Can you work these out from the model? Positions are in its coordinate system, mm. Give positions to 0.01 mm unless a question says otherwise; leave off trailing zeros. Order: outer loops, then holes, each group sorted by start corner. A loop starts at its lowest first (then second) coordinate and runs counter-clockwise, first axis right, second up.
Item 1: I want a section at B-B, the plane z = 3. Write out the boundary of the cut face in (x, y), then the cut area to 3 significant figures.
Item 2: If I drill on line 1 along Z through (x, y) = (0, -15) (3 decimals); line 2 along X through (y, z) = (-9, 9.5); line 3 along Z through (x, y) = (1.5, -6.5) (3 decimals), over which ranges is the centre line in solid material (lowest first)?
Item 3: I want a section at A-A, the plane y = -15. Write out the boundary of the cut face in (x, z) (1 decimal).
Item 4: I want a section at C-C, the plane x = 2. Write out the boundary of the cut face in (y, z) (3 decimals).
Item 5: I'm going to push flat-ended pins straight in: pin 1 Ø3 at (x, z) = (-11, 10) entering from +Y; pin 2 Ø10 at (x, z) = (0, 10.795) entering from -Y. Where does each tip first touch, or does it pass through?
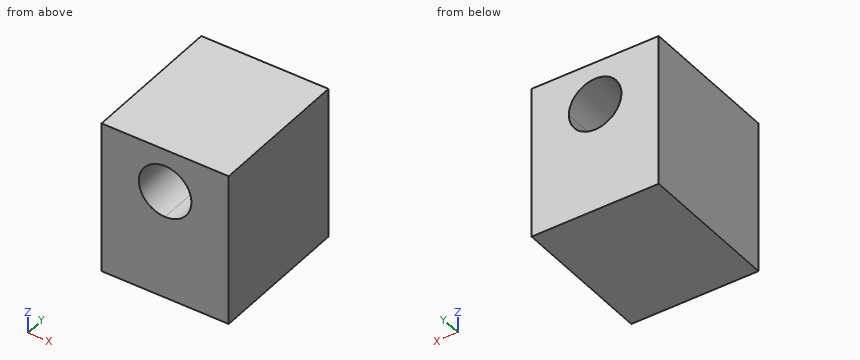
```python
from build123d import *

# Parameters (mm, degrees)
F0_W     = 41.275
F0_H     = 49.53
F1_DEPTH = 46.99


with BuildPart() as f1:
    # F0 (on Front) → F1 (new body)
    with BuildSketch(Plane.XZ):
        Rectangle(F0_W, F0_H)
        with BuildLine():
            ThreePointArc((0, 2.266854), (-6.03031, 16.82531), (8.528146, 10.795))
            ThreePointArc((8.528146, 10.795), (6.03031, 4.76469), (0, 2.266854))
        make_face(mode=Mode.SUBTRACT)
    extrude(amount=F1_DEPTH)


solid = f1.part
```
Results list:
1. outline: (-20.64, -46.99) - (-3.46, -46.99) - (-3.46, 0) - (-20.64, 0) - close; (3.46, -46.99) - (20.64, -46.99) - (20.64, 0) - (3.46, 0) - close
1. area: 1,610 mm2
2. line 1: z = -24.765 to 2.267, 19.323 to 24.765
2. line 2: x = -20.64 to -8.43, 8.43 to 20.64
2. line 3: z = -24.765 to 2.4, 19.19 to 24.765
3. outline: (-20.6, -24.8) - (20.6, -24.8) - (20.6, 24.8) - (-20.6, 24.8) - close; hole circle Ø17.1 at (0, 10.8)
4. outline: (-46.99, -24.765) - (0, -24.765) - (0, 2.505) - (-46.99, 2.505) - close; (-46.99, 19.085) - (0, 19.085) - (0, 24.765) - (-46.99, 24.765) - close
5. pin 1: stops at y = 0
5. pin 2: passes through
